For this review, take the finished solid that the model builds, in its own axes (mm). Coordinates: 2 decimals unless noted, no trailing zeros. Write each loop counter-clockwise with the first axis right and the second up, starting at its lowest first coordinate (ties: lowest second). Pieces come first, ordered by that corner, then holes. Notation, with made-up numbers: (17.25, 55) -> (61.25, 55) arc R23 ccw to (61.25, 89) -> close; hole circle Ø8 at (54, 11.25). An arc over 180 degrees is marked (long way). Put each result on its own line as item: value. Start each with the question number.
Item 1: Consider section B-B on z = 7. Give the boundary of the cut face in (x, y).
Item 2: Insertion check: P1, Ø10, axis at y = -43, z = 8, coming from the +X side; P2, Ø1.5, axis at y = -114, z = 12.5, coming from the -X side; P3, Ø8, axis at y = -149, z = 8.5, coming from the -X side. Each pin has a flat end and moves straight along its axis. Give the tip position at first contact, or say it passes through.
Item 3: The part is to be moulded in two halves that separate along X. For faces 1 (the flat face through (2.296, -98.6, 10.276)), 2 (the cylindrical face through (42.99, -101.4, 1.21)), 3 (the cylindrical face through (24.801, -98.6, 16.473)), 4 (the flat face through (24, -99, 0)), say which applies: +X half, -X half, draft (parallel to the pull), parting line (faces both ways), or undercut.
Item 4: To check wall thickness, follow L1, parallel to Z at x = 37, y = -71.5; L2, parallel to Z at x = 13, y = -129; L3, parallel to X at y = -81.5, z = 1.75. State the ranges of each line that lie inside material, in increasing order.
Item 5: Consider section C-C on x = 31. Give the boundary of the cut face in (y, z), and give its area (3 significant figures).
Item 6: Consider section A-A on y = -136. Give the boundary of the cut face in (x, z), and give its area (3 significant figures).
```python
from build123d import *

# Parameters (mm, degrees)
F1_DEPTH = 200
F2_R     = 6
F3_R     = 2


with BuildPart() as f1:
    # F0 (on Front) → F1 (new body)
    with BuildSketch(Plane.XZ):
        with BuildLine():
            Line((0, 19), (5, 0))
            Line((5, 0), (44, 0))
            Line((44, 0), (49, 19))
            ThreePointArc((49, 19), (24.5, 16.472337), (0, 19))
        make_face()
    extrude(amount=F1_DEPTH)

    # F2
    f2_edges = [f1.edges().sort_by_distance(p)[0] for p in [
        (5, -100, 0),
        (44, -100, 0),
    ]]
    fillet(f2_edges, radius=F2_R)

    # F3
    f3_edges = [f1.edges().sort_by_distance(p)[0] for p in [
        (49, -100, 19),
        (0, -100, 19),
    ]]
    fillet(f3_edges, radius=F3_R)


solid = f1.part
```
Return value:
1. outline: (3.16, -200) -> (45.84, -200) -> (45.84, 0) -> (3.16, 0) -> close
2. P1: x = 47.42
2. P2: x = 1.51
2. P3: x = 1.71
3. face 1: -X half
3. face 2: +X half
3. face 3: undercut
3. face 4: draft
4. L1: 0 to 17.13
4. L2: 0 to 17.02
4. L3: 5.39 to 43.61
5. outline: (-200, 0) -> (0, 0) -> (0, 16.65) -> (-200, 16.65) -> close
5. area: 3,330 mm^2
6. outline: (0.81, 15.92) -> (3.82, 4.47) arc R6 ccw to (9.63, 0) -> (39.37, 0) arc R6 ccw to (45.18, 4.47) -> (48.19, 15.92) arc R2 ccw to (45.9, 18.4) arc R120 cw to (3.1, 18.4) arc R2 ccw to start
6. area: 740 mm^2
